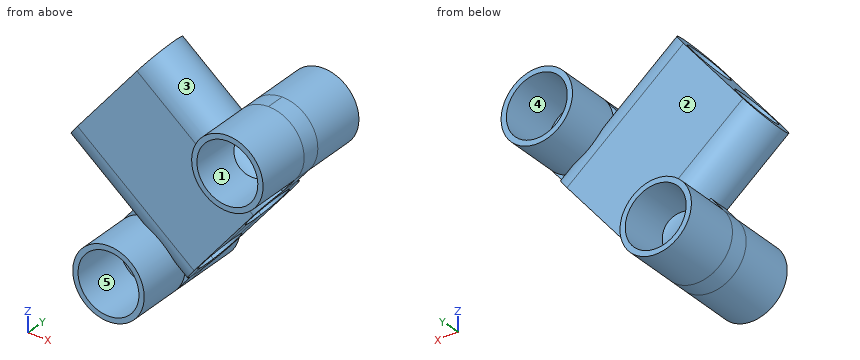
from build123d import *
from build123d.topology import SkipClean

# Parameters (mm, degrees)
BOSS_EXTRUDE2_DEPTH      = 5
BOSS_EXTRUDE3_DEPTH      = 15
BOSS_EXTRUDE3_DEPTH_BACK = 20
SKETCH4_R                = 9.5
SKETCH4_R_2              = 8.1
BOSS_EXTRUDE4_DEPTH      = 21
BOSS_EXTRUDE4_DEPTH_BACK = 19
SKETCH5_R                = 6.1
CUT_EXTRUDE2_START       = -41
SKETCH6_R                = 6.1
CUT_EXTRUDE2_DEPTH       = 41


with BuildPart() as part:
    # Sketch3 → Boss-Extrude2 (new body)
    with BuildSketch(Plane(origin=(0, 0, 0), x_dir=(1, 0, 0), z_dir=(0, 1, 0))):
        with BuildLine():
            Line((-3.174904091, 31.814719718), (28.442244127, -6.919708618))
            ThreePointArc((28.442244127, -6.919708618), (27.089960905, -20.286508163), (13.723161359, -18.934224941))
            Line((13.723161359, -18.934224941), (-17.893986859, 19.800203396))
            ThreePointArc((-17.893986859, 19.800203396), (-16.541703636, 33.167002941), (-3.174904091, 31.814719718))
        make_face()
    extrude(amount=BOSS_EXTRUDE2_DEPTH)

    # Sketch4 → Boss-Extrude3 (add, two sides: drawn at the far end of the back side and taken through both)
    # profile 1 of 2: a face of its own
    with SkipClean():  # the faces are left unmerged after this step: merging them gives an invalid solid
        with BuildSketch(Plane(origin=(0, 5, 0), x_dir=(1, 0, 0), z_dir=(0, 1, 0)).offset(-BOSS_EXTRUDE3_DEPTH_BACK)):
            with Locations(Location((-10.534445475, 25.807461557, 0), (0, 0, 270))):
                Circle(SKETCH4_R)
            with Locations(Location((-10.534445475, 25.807461557, 0), (0, 0, 270))):
                Circle(SKETCH4_R_2, mode=Mode.SUBTRACT)
        # profile 2 of 2: a face of its own
        with BuildSketch(Plane(origin=(0, 5, 0), x_dir=(1, 0, 0), z_dir=(0, 1, 0)).offset(-BOSS_EXTRUDE3_DEPTH_BACK)):
            with Locations(Location((21.082702743, -12.92696678, 0), (0, 0, 270))):
                Circle(SKETCH4_R)
            with Locations(Location((21.082702743, -12.92696678, 0), (0, 0, 270))):
                Circle(SKETCH4_R_2, mode=Mode.SUBTRACT)
        extrude(amount=BOSS_EXTRUDE3_DEPTH + BOSS_EXTRUDE3_DEPTH_BACK)
    add(part.part.scale(1), mode=Mode.REPLACE)  # the faces are merged on a copy

    # Sketch5 → Boss-Extrude4 (add, two sides: drawn at the far end of the back side and taken through both)
    with BuildSketch(Plane(origin=(-1.03943662, 0, 0.848444732), x_dir=(0.6323429643622943, 0, 0.774688566729564), z_dir=(-0.774688566729564, 0, 0.6323429643622943)).offset(-BOSS_EXTRUDE4_DEPTH_BACK)):
        with BuildLine():
            Line((-14.154127884, 9.71687123), (10.845872116, 9.71687123))
            ThreePointArc((10.845872116, 9.71687123), (18.062743346, 2.5), (10.845872116, -4.71687123))
            Line((10.845872116, -4.71687123), (-14.154127884, -4.71687123))
            ThreePointArc((-14.154127884, -4.71687123), (-21.370999114, 2.5), (-14.154127884, 9.71687123))
        make_face()
        with Locations((-11.654127884, 2.5)):
            Circle(SKETCH5_R, mode=Mode.SUBTRACT)
        with Locations((8.345872116, 2.5)):
            Circle(SKETCH5_R, mode=Mode.SUBTRACT)
    extrude(amount=BOSS_EXTRUDE4_DEPTH + BOSS_EXTRUDE4_DEPTH_BACK)

    # Sketch6 → Cut-Extrude2 (cut)
    with BuildSketch(Plane(origin=(-17.307896522, 0, 14.127646984), x_dir=(0.6323429643622943, 0, 0.774688566729564), z_dir=(-0.774688566729564, 0, 0.6323429643622943)).offset(CUT_EXTRUDE2_START)):
        with Locations((-11.654127884, 2.5)):
            Circle(SKETCH6_R)
        with Locations((8.345872116, 2.5)):
            Circle(SKETCH6_R)
    extrude(amount=CUT_EXTRUDE2_DEPTH, mode=Mode.SUBTRACT)


solid = part.part
Design review of the part built by this model. Coordinates are the model's own, in mm. Face numbers are marked on the shaded views. A direction names the side the tool comes from. Coordinates: 2 decimals unless noted, no trailing zeros. Loops run counter-clockwise (first coordinate to the right, second up) from the corner with the lowest first, then second, coordinate; pieces in that order, holes last.
Item 1: For the marked faces 3, 4 and 5, list the 3-axis set-ups (+Z, -Z, +X, -X, +Y, -Y) from which the entire face can be reached by the end or side of a thin tool; tool diameter is ignored.
Completed:
face 3: none
face 4: +Y
face 5: -Y
Item 2: Add section A-A (y = 4). Write out the cut boundary in (x, z).
Completed:
outline: (-30.72, -2.31) - (-14.45, -15.59) - (-17.89, -19.8) arc R9.5 ccw to (-3.17, -31.81) - (2.57, -24.77) - (-28.42, 0.52) - close; (-20.94, 9.68) - (10.05, -15.61) - (15.22, -9.28) - (-15.77, 16.01) - close; (-8.29, 25.17) - (22.7, -0.12) - (28.44, 6.92) arc R9.5 ccw to (13.72, 18.93) - (10.28, 14.72) - (-5.99, 28) - close
Item 3: Clearance check with flat-ended pins moving along their axes: pin 1 (9.5 mm diameter, centred on x = 21.08, z = 12.93, fed in from -Y); pin 2 (10 mm diameter, centred on x = -19.5, y = -0.5, fed in from +Z); pin 3 (1 mm diameter, centred on y = -5, z = 17, fed in from -X). State where each tip first meets the part, or that it passes through.
Completed:
pin 1: stops at y = 0
pin 2: stops at z = 17.32
pin 3: stops at x = -15.3
Item 4: Add section B-B (z = -30.5). Write out the cut boundary in (x, y), and give its area (3 significant figures).
Completed:
outline: (-18.79, -15) - (-17.14, -15) - (-17.14, 0) - (-3.93, 0) - (-3.93, -15) - (-2.27, -15) - (-2.27, 0) - (-2.1, 0) - (-2.1, 5) - (-2.27, 5) - (-2.27, 20) - (-3.93, 20) - (-3.93, 5) - (-17.14, 5) - (-17.14, 20) - (-18.79, 20) - close
area: 183 mm2
Item 5: Draft analysis for pull direction X (two halves, no side actions). For the marked faces 1 and 2, state which applies: pulls with the +X half, pulls with the -X half, needs draft (parallel to the pull), parting line crosses it, or undercut.
Completed:
face 1: undercut
face 2: needs draft
Item 6: Wall thickness on L1, parallel to Z at x = -6, y = 3.5; L2, parallel to X at y = 7, z = -4.5; L3, parallel to Z at x = 27.5, y = -7: over which ranges is each line inside the solid? List them lowest first.
Completed:
L1: z = -34.16 to -17.91, -2.38 to 7.9, 23.44 to 27.98
L2: x = -25.79 to -19.43, -6.4 to 12.2
L3: z = 5.92 to 7.98, 17.87 to 19.93
Item 7: Add section C-C (x = 1.5). Give the number of separate pieces and of enclosed holes in the cut face, and give its area (3 significant figures).
Completed:
separate pieces: 1
enclosed holes: 2
area: 356 mm2
